Here's how the part is built. I have some questions about the finished solid (model axes, mm). Face numbers are marked on the shaded views. A direction names the side the tool comes from. Give positions to 0.01 mm unless a question says otherwise; leave off trailing zeros. Write each loop counter-clockwise with the first axis right and the second up, starting at its lowest first coordinate (ties: lowest second). Pieces come first, ordered by that corner, then holes. Notation, with made-up numbers: (61, 10) - (89, 10) arc R26 ccw to (89, 32) - close; hole circle Ø4 at (23, 60). An arc over 180 degrees is marked (long way). Write each question's results on one line, items separated by ' | '. Start each with the question number.
Item 1: We'd pull the mould along Y, two halves only. Please class the marked faces 1, 2 and 3: +Y half, -Y half, draft (parallel to the pull), parting line (faces both ways), or undercut.
Item 2: Suppose I cut it at C-C on x = -22. List the corners of the cut face in (y, z) for me, then the cut area to 3 significant figures.
Item 3: Will these pins go through, and if not, where does the flat tip stop? P1, Ø16, axis at y = -17, z = 1, coming from the +X side (3 decimals); P2, Ø6, axis at y = -38.5, z = -14, coming from the +X side; P3, Ø25, axis at x = -7, z = -36, coming from the -Y side.
Item 4: Suppose I cut it at A-A on y = -20. List the corners of the cut face in (x, z) for me.
Item 5: Suppose I cut it at B-B on z = 43. List the corners of the cut face in (x, y) for me, then the cut area to 3 significant figures.
Item 6: Please list where these lines run through material, in increasing order: line 1 along X through (y, z) = (-32, 12); line 2 along Y through (x, z) = (11.5, -62); line 3 along X through (y, z) = (-37, 12).
Item 7: Suppose I cut it at D-D on y = -37. List the corners of the cut face in (x, z) for me, then the cut area to 3 significant figures.
Item 8: Which directions (+Z, -Z, +X, -X, +Y, -Y) give clear straight access to the entire face, cutting with the end or side of a thin tool? Please do the marked faces 4 and 5.
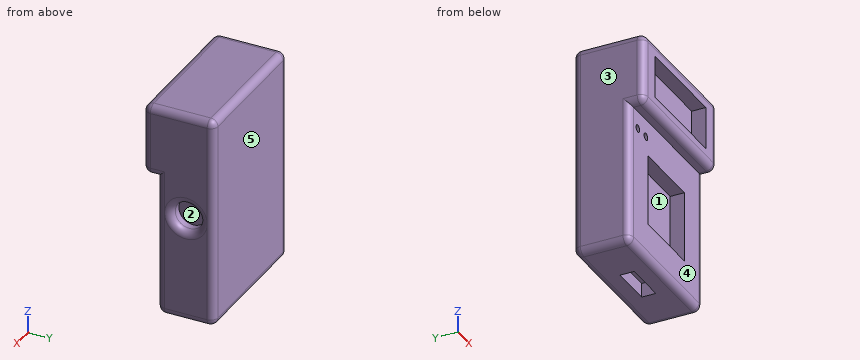
```python
from build123d import *

# Parameters (mm, degrees)
F0_W      = 100
F0_H      = 50
F1_DEPTH  = 50
F3_DEPTH  = 10
F0_H_2    = 100
F4_DEPTH  = 40
F5_R      = 10
F6_DEPTH  = 10
F7_W      = 70
F7_H      = 30
F8_DEPTH  = 10
F9_W      = 30
F9_H      = 10
F10_DEPTH = 10
F11_W     = 50
F11_H     = 50
F12_DEPTH = 10
F13_R     = 4.99999
F14_R     = 2.5
F15_DEPTH = 10


# Not quite as in the source:
# - a fillet or chamfer is up to 0.001 mm smaller than in the source, because OpenCascade refuses the exact size


with BuildPart() as f1:
    # F0 (on Front) → F1 (new body)
    with BuildSketch(Plane.XZ):
        with Locations((0, 50)):
            Rectangle(F0_W, F0_H)
    extrude(amount=F1_DEPTH)

    # F2 (on face) → F3 (cut)
    with BuildSketch(Plane.YZ.offset(50)):
        with BuildLine():
            Line((-35, 25), (-15, 25))
            ThreePointArc((-15, 25), (-25, 35), (-35, 25))
        make_face()
        with BuildLine():
            ThreePointArc((-35, 25), (-25, 15), (-15, 25))
            Line((-15, 25), (-35, 25))
        make_face()
    extrude(amount=-F3_DEPTH, mode=Mode.SUBTRACT)

    # F0 (on Front) → F4 (join)
    with BuildSketch(Plane.XZ):
        with Locations((0, 50)):
            Rectangle(F0_W, F0_H)
        with Locations((0, -25)):
            Rectangle(F0_W, F0_H_2)
    extrude(amount=F4_DEPTH)

    # F5 (on face) → F6 (cut)
    with BuildSketch(Plane.YZ.offset(50)):
        with Locations((-20, 0)):
            Circle(F5_R)
    extrude(amount=-F6_DEPTH, mode=Mode.SUBTRACT)

    # F7 (on face) → F8 (cut)
    with BuildSketch(Plane.XZ.offset(50)):
        with Locations((0, 50)):
            Rectangle(F7_W, F7_H)
    extrude(amount=-F8_DEPTH, mode=Mode.SUBTRACT)

    # F9 (on face) → F10 (cut)
    with BuildSketch(Plane(origin=(0, 0, -75), x_dir=(1, 0, 0), z_dir=(0, 0, -1))):
        with Locations((0, 20)):
            Rectangle(F9_W, F9_H)
    extrude(amount=-F10_DEPTH, mode=Mode.SUBTRACT)

    # F11 (on face) → F12 (cut)
    with BuildSketch(Plane.XZ.offset(40)):
        with Locations((0, -25)):
            Rectangle(F11_W, F11_H)
    extrude(amount=-F12_DEPTH, mode=Mode.SUBTRACT)

    # F13 (radius 5 in the source; OpenCascade refuses exactly that, so slightly less here)
    f13_edges = [f1.edges().sort_by_distance(p)[0] for p in [
        (0, -50, 75),
        (-50, -50, 50),
        (50, -50, 50),
        (0, -50, 25),
        (-50, -40, -25),
        (50, -40, -25),
        (0, -40, -75),
        (0, 0, 75),
        (-50, 0, 0),
        (50, -25, 75),
        (-50, -25, 75),
        (50, 0, 0),
        (50, -20, -75),
        (50, -45, 25),
        (50, -30, 0),
        (0, 0, -75),
        (-50, -20, -75),
        (-50, -45, 25),
    ]]
    fillet(f13_edges, radius=F13_R)

    # F14 (on face) → F15 (cut)
    with BuildSketch(Plane.XZ.offset(40)):
        with Locations((-39.3138879017, 12.5)):
            Circle(F14_R)
        with Locations((-28.179211659, 12.5)):
            Circle(F14_R)
    extrude(amount=-F15_DEPTH, mode=Mode.SUBTRACT)


solid = f1.part
```
Checked values:
1) face 1: -Y half | face 2: undercut | face 3: draft
2) outline: (-50, 30) arc R5 ccw to (-45, 25) - (-40, 25) - (-40, 0) - (-30, 0) - (-30, -50) - (-40, -50) - (-40, -70) arc R5 ccw to (-35, -75) - (-5, -75) arc R5 ccw to (0, -70) - (0, 70) arc R5 ccw to (-5, 75) - (-45, 75) arc R5 ccw to (-50, 70) - (-50, 65) - (-40, 65) - (-40, 35) - (-50, 35) - close | area: 5,670 mm^2
3) P1: stops at x = 48.205 | P2: stops at x = 49.97 | P3: stops at y = -30
4) outline: (-50, -70) arc R5 ccw to (-45, -75) - (-15, -75) - (-15, -65) - (15, -65) - (15, -75) - (45, -75) arc R5 ccw to (50, -70) - (50, -15) arc R5 ccw to (45, -10) - (40, -10) - (40, 10) - (45, 10) arc R5 ccw to (50, 15) - (50, 70) arc R5 ccw to (45, 75) - (-45, 75) arc R5 ccw to (-50, 70) - close
5) outline: (-50, -45) arc R5 ccw to (-45, -50) - (-35, -50) - (-35, -40) - (35, -40) - (35, -50) - (45, -50) arc R5 ccw to (50, -45) - (50, -5) arc R5 ccw to (45, 0) - (-45, 0) arc R5 ccw to (-50, -5) - close | area: 4,280 mm^2
6) line 1: x = -50 to -41.76, -36.86 to -30.63, -25.73 to 50 | line 2: y = -40 to 0 | line 3: x = -49.58 to -41.76, -36.86 to -30.63, -25.73 to 49.58
7) outline: (-50, 30) arc R5 ccw to (-49.58, 28) - (-49.58, -70) arc R4.58 ccw to (-45, -74.58) - (45, -74.58) arc R4.58 ccw to (49.58, -70) - (49.58, 28) arc R5 ccw to (50, 30) - (50, 70) arc R5 ccw to (45, 75) - (-45, 75) arc R5 ccw to (-50, 70) - close; hole circle Ø5 at (-39.31, 12.5); hole circle Ø5 at (-28.18, 12.5); hole (-25, -50) - (25, -50) - (25, 0) - (-25, 0) - close | area: 12,300 mm^2
8) face 4: -Z, +X, -X, -Y | face 5: +Z, -Z, +X, -X, +Y
